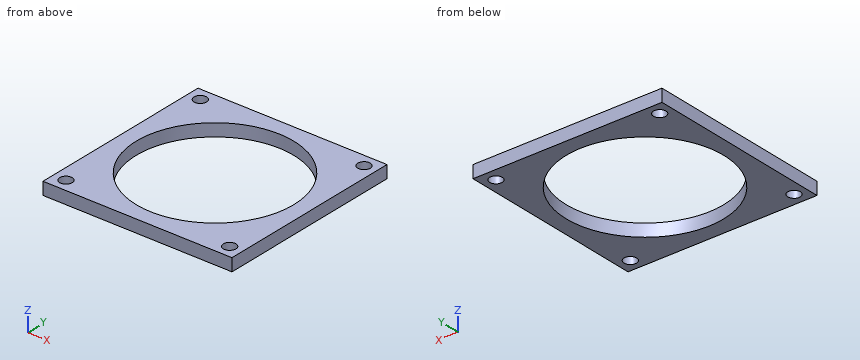
```python
from build123d import *

# Parameters (mm, degrees)
SKETCH1_W               = 38.1
SKETCH1_H               = 38.1
BOSS_EXTRUDE1_DEPTH     = 2.54
CUT_EXTRUDE1_DEPTH      = 28.060240206
CUT_EXTRUDE1_DEPTH_BACK = 28.060240206
SKETCH2_R               = 15.875
HOLE1_OUTLINE_R         = 1.27
HOLE1_DEPTH             = 2.54


# Read off the part's stored shape, not the designer's step: Hole1
with BuildPart() as part:
    # Sketch1 → Boss-Extrude1 (new body)
    with BuildSketch(Plane.XY):
        Rectangle(SKETCH1_W, SKETCH1_H)
    extrude(amount=BOSS_EXTRUDE1_DEPTH)

    # Sketch2 → Cut-Extrude1 (cut, two sides: drawn at the far end of the back side and taken through both)
    with BuildSketch(Plane.XY.offset(2.54).offset(-CUT_EXTRUDE1_DEPTH_BACK)):
        Circle(SKETCH2_R)
    extrude(amount=CUT_EXTRUDE1_DEPTH + CUT_EXTRUDE1_DEPTH_BACK, mode=Mode.SUBTRACT)

    # Hole1 outline → Hole1 (cut)
    with BuildSketch(Plane.XY):
        with Locations((-16.51, 16.51)):
            Circle(HOLE1_OUTLINE_R)
        with Locations((16.51, 16.51)):
            Circle(HOLE1_OUTLINE_R)
        with Locations((16.51, -16.51)):
            Circle(HOLE1_OUTLINE_R)
        with Locations((-16.51, -16.51)):
            Circle(HOLE1_OUTLINE_R)
    extrude(amount=HOLE1_DEPTH, mode=Mode.SUBTRACT)


solid = part.part
```
Can you work these out from the model? Positions are in its coordinate system, mm. Round coordinates to 2 decimals unless told otherwise and drop trailing zeros. Loops run counter-clockwise (first coordinate to the right, second up) from the corner with the lowest first, then second, coordinate; pieces in that order, holes last. Notation, with made-up numbers: (3.25, 60.25) -> (55.25, 60.25) arc R28 ccw to (55.25, 85.25) -> close; hole circle Ø7 at (33.25, 80.5). An arc over 180 degrees is marked (long way). Answer in a Markdown table with one row per item.
Item 1: Suppose I cut it at C-C, the plane z = 1.75. List the corners of the cut face in (x, y) for me (3 decimals).
Answer block:
| item | result |
|---|---|
| outline | (-19.05, -19.05) -> (19.05, -19.05) -> (19.05, 19.05) -> (-19.05, 19.05) -> close; hole circle Ø2.54 at (-16.51, -16.51); hole circle Ø2.54 at (-16.51, 16.51); hole circle Ø31.75 at (0, 0); hole circle Ø2.54 at (16.51, -16.51); hole circle Ø2.54 at (16.51, 16.51) |
Item 2: Suppose I cut it at D-D, the plane y = 16.51. List the corners of the cut face in (x, z) for me, plus the area to 3 significant figures.
Answer block:
| item | result |
|---|---|
| outline | (-19.05, 0) -> (-17.78, 0) -> (-17.78, 2.54) -> (-19.05, 2.54) -> close; (-15.24, 0) -> (15.24, 0) -> (15.24, 2.54) -> (-15.24, 2.54) -> close; (17.78, 0) -> (19.05, 0) -> (19.05, 2.54) -> (17.78, 2.54) -> close |
| area | 83.9 mm² |
Item 3: Suppose I cut it at A-A, the plane y = 0. List the corners of the cut face in (x, z) for me (3 decimals).
Answer block:
| item | result |
|---|---|
| outline | (-19.05, 0) -> (-15.875, 0) -> (-15.875, 2.54) -> (-19.05, 2.54) -> close; (15.875, 0) -> (19.05, 0) -> (19.05, 2.54) -> (15.875, 2.54) -> close |
Item 4: Will these pins go through, and if not, where does the flat tip stop? P1, Ø2, axis at x = 16.51, y = -16.51, coming from the +Z side; P2, Ø4, axis at x = -16.51, y = 16.51, coming from the +Z side.
Answer block:
| item | result |
|---|---|
| P1 | through |
| P2 | z = 2.54 |
Item 5: If I drill on probe 1 along Y at (x, z) = (-16.51, 1); probe 2 along X at (y, z) = (16, 0.5); probe 3 along Y at (x, z) = (17.5, 0.55), over which ranges is the centre line in solid material (lowest first)?
Answer block:
| item | result |
|---|---|
| probe 1 | -19.05 to -17.78, -15.24 to 15.24, 17.78 to 19.05 |
| probe 2 | -19.05 to -17.67, -15.35 to 15.35, 17.67 to 19.05 |
| probe 3 | -19.05 to -17.31, -15.71 to 15.71, 17.31 to 19.05 |
